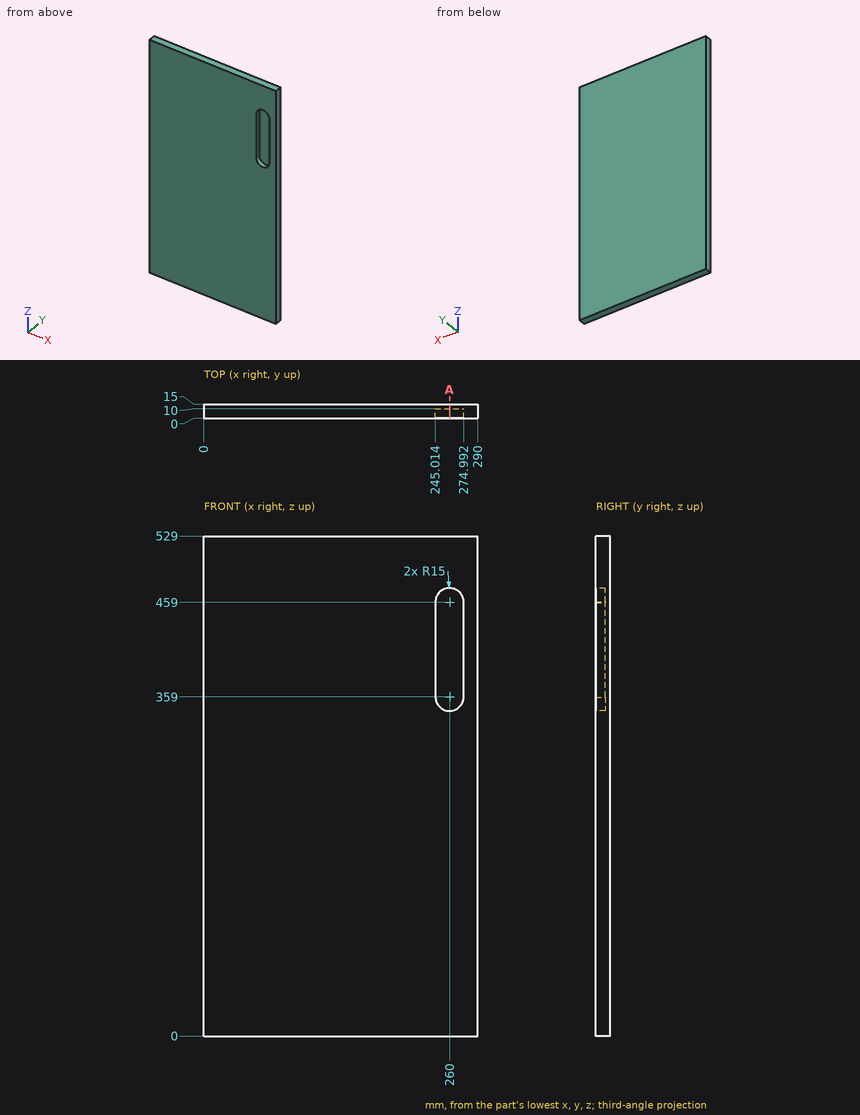
Drawing for the job (mm, zero at the part's lowest x, y, z). Round coordinates to 2 decimals unless told otherwise and drop trailing zeros. Write each loop counter-clockwise with the first axis right and the second up, starting at its lowest first coordinate (ties: lowest second). Pieces come first, ordered by that corner, then holes. Notation, with made-up numbers: (1.5, 61) - (30.5, 61) arc R12 ccw to (30.5, 81) - close; hole circle Ø3 at (87.5, -34). An arc over 180 degrees is marked (long way). Use CSV: the item, a comma, the result in double quotes.
(1) Pin check, flat tip, straight feed: P1, Ø9, axis at x = 267, z = 432.5, coming from the -Y side. Stop position of the tip, or through.
Response:
P1,"y = 10"
(2) Wall check: line 1 (X direction, y = 8.25, z = 422) (1 decimal); line 2 (X direction, y = 4, z = 356); line 3 (Z direction, x = 250, y = 3.25). Give the ranges that are in metal, low to high.
Response:
line 1,"0 to 245, 275 to 290"
line 2,"0 to 245.3, 274.7 to 290"
line 3,"0 to 347.82, 470.18 to 529"
(3) Band-saw the part on A-A (x = 260). Write the cut outline in (y, z).
Response:
outline,"(0, 0) - (15, 0) - (15, 529) - (0, 529) - (0, 474) - (10, 474) - (10, 344) - (0, 344) - close"
